The listing builds one solid part. Answer for the finished solid, in the listing's coordinates (mm). Coordinates: 2 decimals unless noted, no trailing zeros. Loops run counter-clockwise (first coordinate to the right, second up) from the corner with the lowest first, then second, coordinate; pieces in that order, holes last. Notation, with made-up numbers: M 88,-36.5 L 103,-36.5 A21 cw 103,2.5 Z; hole C 56,76 d10. An arc over 180 degrees is marked long. Answer as a JSON object with one key per item and string values. Group by question number.
1. A cutting plane is placed at C-C on z = -2.54. Give the vertices of the cut face in (x, y).
2. A cutting plane is placed at A-A on x = -0.6. Give the vertices of the cut face in (y, z).
3. Straight lines are drawn through the part: L1, parallel to Z at x = 0, y = 4; L2, parallel to Z at x = 0.55, y = 4.5; L3, parallel to X at y = 1, z = -7. For each, find the intervals that lie inside material, in ascending order.
4. A cutting plane is placed at D-D on z = -5.5. Give the vertices of the cut face in (x, y).
5. A cutting plane is placed at B-B on y = 1.75. Give the vertices of the cut face in (x, z).
6. Given pin 1 (1.6 mm diameter, centred on x = 0, z = 0, fed in from +Y), flat-ended and moving along its own axis, determine where the tip first touches the part or whether it passes through.
Autodesk Inventor part; units mm, degrees
ref_plane "YZ Plane" through (0, 0, 0) normal (1, 0, 0) x (0, 1, 0)
ref_plane "XZ Plane" through (0, 0, 0) normal (0, 1, 0) x (-1, 0, 0)
ref_plane "XY Plane" through (0, 0, 0) normal (0, 0, 1) x (1, 0, 0)
sketch "Sketch1" plane through (0, 0, 0) normal (0, 1, 0) x (-1, 0, 0)
  circle A0 centre (0, 0) radius 1
  line L0 (2, 2) -> (-2, 2)
  line L1 (-2, 2) -> (-2, -12.16)
  line L2 (-2, -12.16) -> (2, -12.16)
  line L3 (2, -12.16) -> (2, 2)
  circle A1 centre (0, -2.54) radius 1
  circle A2 centre (0, -5.08) radius 1
  circle A3 centre (0, -7.62) radius 1
  circle A4 centre (0, -10.16) radius 1
  dimension "d0" = 2
  dimension "d3" = 2.54
  dimension "d8" = 1
  dimension "d9" = 1
  dimension "d10" = 1
  dimension "d11" = 1
extrude "Extrusion1" add sketch "Sketch1" along normal blind 12.5
equation "\"d9\" = d8"
equation "\"d10\" = d8"
equation "\"d11\" = d8"
properties part number "Encoder Header Spacer 2"
From the geometry:
{
 "1": {"outline": "M -2,0 L -1,0 L -1,12.5 L -2,12.5 Z; M 1,0 L 2,0 L 2,12.5 L 1,12.5 Z"},
 "2": {"outline": "M 0,-12.16 L 12.5,-12.16 L 12.5,-10.96 L 0,-10.96 Z; M 0,-9.36 L 12.5,-9.36 L 12.5,-8.42 L 0,-8.42 Z; M 0,-6.82 L 12.5,-6.82 L 12.5,-5.88 L 0,-5.88 Z; M 0,-4.28 L 12.5,-4.28 L 12.5,-3.34 L 0,-3.34 Z; M 0,-1.74 L 12.5,-1.74 L 12.5,-0.8 L 0,-0.8 Z; M 0,0.8 L 12.5,0.8 L 12.5,2 L 0,2 Z"},
 "3": {"L1": "z = -12.16 to -11.16, -9.16 to -8.62, -6.62 to -6.08, -4.08 to -3.54, -1.54 to -1, 1 to 2", "L2": "z = -12.16 to -11, -9.32 to -8.46, -6.78 to -5.92, -4.24 to -3.38, -1.7 to -0.84, 0.84 to 2", "L3": "x = -2 to -0.78, 0.78 to 2"},
 "4": {"outline": "M -2,0 L -0.91,0 L -0.91,12.5 L -2,12.5 Z; M 0.91,0 L 2,0 L 2,12.5 L 0.91,12.5 Z"},
 "5": {"outline": "M -2,-12.16 L 2,-12.16 L 2,2 L -2,2 Z; hole C 0,-10.16 d2; hole C 0,-7.62 d2; hole C 0,-5.08 d2; hole C 0,-2.54 d2; hole C 0,0 d2"},
 "6": {"pin 1": "passes through"}
}
